```python
from build123d import *

# Parameters (mm, degrees)
SKETCH_1_R      = 37.5
SKETCH_1_R_2    = 4
EXTRUDE_1_DEPTH = 1


with BuildPart() as part:
    # 草图1 → 凸台-拉伸1 (new body)
    with BuildSketch(Plane(origin=(0, 0, 0), x_dir=(1, 0, 0), z_dir=(0, 1, 0))):
        with BuildLine():
            Line((18.734993995, 57), (-18.734993995, 57))
            ThreePointArc((-18.734993995, 57), (-59.736901958, -5.612712749), (-7.789712862, -59.4921875))
            ThreePointArc((-7.789712862, -59.4921875), (0, -55), (7.789712862, -59.4921875))
            ThreePointArc((7.789712862, -59.4921875), (59.736901958, -5.612712749), (18.734993995, 57))
        make_face()
        with Locations(Location((0, 0, 0), (0, 0, 270))):
            Circle(SKETCH_1_R, mode=Mode.SUBTRACT)
        with Locations(Location((-48.041735691, 19.899538483, 0), (0, 0, 270))):
            Circle(SKETCH_1_R_2, mode=Mode.SUBTRACT)
        with Locations(Location((-19.899538483, 48.041735691, 0), (0, 0, 270))):
            Circle(SKETCH_1_R_2, mode=Mode.SUBTRACT)
        with Locations(Location((19.899538483, 48.041735691, 0), (0, 0, 270))):
            Circle(SKETCH_1_R_2, mode=Mode.SUBTRACT)
        with Locations(Location((48.041735691, 19.899538483, 0), (0, 0, 270))):
            Circle(SKETCH_1_R_2, mode=Mode.SUBTRACT)
        with Locations(Location((48.041735691, -19.899538483, 0), (0, 0, 270))):
            Circle(SKETCH_1_R_2, mode=Mode.SUBTRACT)
        with Locations(Location((19.899538483, -48.041735691, 0), (0, 0, 270))):
            Circle(SKETCH_1_R_2, mode=Mode.SUBTRACT)
        with Locations(Location((-19.899538483, -48.041735691, 0), (0, 0, 270))):
            Circle(SKETCH_1_R_2, mode=Mode.SUBTRACT)
        with Locations(Location((-48.041735691, -19.899538483, 0), (0, 0, 270))):
            Circle(SKETCH_1_R_2, mode=Mode.SUBTRACT)
    extrude(amount=EXTRUDE_1_DEPTH)


solid = part.part
```
Verification items for the finished model (mm, model axes). Coordinates: 2 decimals unless noted, no trailing zeros. Loops run counter-clockwise (first coordinate to the right, second up) from the corner with the lowest first, then second, coordinate; pieces in that order, holes last. Notation, with made-up numbers: (-33.75, 86) -> (-26.75, 86) arc R26 ccw to (-26.75, 112) -> close; hole circle Ø7 at (56, 89). An arc over 180 degrees is marked (long way). Answer in a Markdown table with one row per item. Add a question column.
1. Section check B-B, the plane z = 0. Enter the section's corners in (x, y).
2. Section check C-C, the plane z = 20. Enter the section's corners in (x, y), then the cut area to 3 significant figures.
3. Section check A-A, the plane x = 0. Enter the section's corners in (y, z), then the cut area to 3 significant figures.
4. Material ranges on probe 1 along X at (y, z) = (0.7, 0); probe 2 along X at (y, z) = (0.25, -49.5); probe 3 along X at (y, z) = (0.8, -21), recorded low to high. Write a range as [from, to].
5. Draft check along Z on faces 1 (the face through (-22.818, 0.493, -29.759)), 2 (the face through (21.101, 0.493, -44.226)), 3 (the face through (-28, 0, 26)), 4 (the face through (-59.83, 0.49, 4.49)). Enter one of: +Z half, -Z half, draft (parallel to the pull), parting line (faces both ways), or undercut.
6. Section check D-D, the plane y = 0.3. Give the number of separate pieces and of enclosed holes in the cut face, then the cut area to 3 significant figures.
7. Depth check by flat-ended pin: P1, Ø7, axis at x = 19.9, z = -48.04, coming from the +Y side. Enter the tip coordinate at first touch or a pass-through.
Derived:
| question | item | result |
|---|---|---|
| 1 | outline | (-60, 0) -> (-37.5, 0) -> (-37.5, 1) -> (-60, 1) -> close; (37.5, 0) -> (60, 0) -> (60, 1) -> (37.5, 1) -> close |
| 2 | outline | (-56.57, 0) -> (-52.04, 0) -> (-52.04, 1) -> (-56.57, 1) -> close; (-44.04, 0) -> (-31.72, 0) -> (-31.72, 1) -> (-44.04, 1) -> close; (31.72, 0) -> (44.04, 0) -> (44.04, 1) -> (31.72, 1) -> close; (52.04, 0) -> (56.57, 0) -> (56.57, 1) -> (52.04, 1) -> close |
| 2 | area | 33.7 mm² |
| 3 | outline | (0, -57) -> (1, -57) -> (1, -37.5) -> (0, -37.5) -> close; (0, 37.5) -> (1, 37.5) -> (1, 55) -> (0, 55) -> close |
| 3 | area | 37.0 mm² |
| 4 | probe 1 | x = [-60, -37.5], [37.5, 60] |
| 4 | probe 2 | x = [-33.91, -23.62], [-16.17, 16.17], [23.62, 33.91] |
| 4 | probe 3 | x = [-56.2, -51.89], [-44.2, -31.07], [31.07, 44.2], [51.89, 56.2] |
| 5 | face 1 | undercut |
| 5 | face 2 | undercut |
| 5 | face 3 | draft |
| 5 | face 4 | parting line |
| 6 | separate pieces | 1 |
| 6 | enclosed holes | 9 |
| 6 | area | 6,360 mm² |
| 7 | P1 | passes through |
